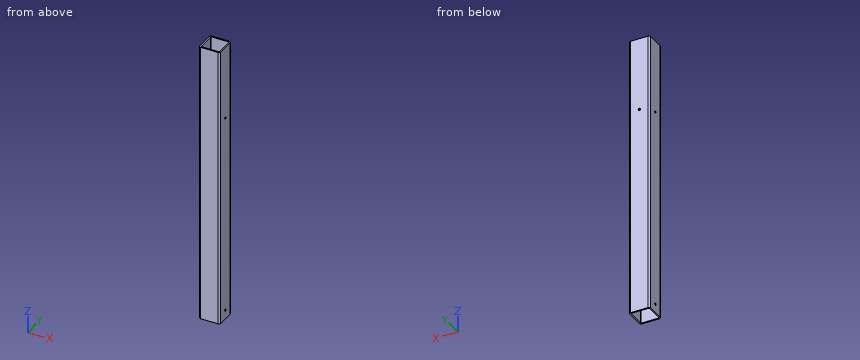
Autodesk Inventor part; units mm, degrees
ref_plane "YZ Plane" through (0, 0, 0) normal (1, 0, 0) x (0, 1, 0)
ref_plane "XZ Plane" through (0, 0, 0) normal (0, 1, 0) x (-1, 0, 0)
ref_plane "XY Plane" through (0, 0, 0) normal (0, 0, 1) x (1, 0, 0)
sketch "Sketch1" plane through (0, 0, 0) normal (0, 0, 1) x (1, 0, 0)
  line L0 (40, 34) -> (40, -34)
  line L1 (34, -40) -> (-34, -40)
  line L2 (-40, -34) -> (-40, 34)
  line L3 (-34, 40) -> (34, 40)
  arc A0 (-34, 40) -> (-40, 34) centre (-34, 34) ccw
  arc A1 (40, 34) -> (34, 40) centre (34, 34) ccw
  arc A2 (34, -40) -> (40, -34) centre (34, -34) ccw
  arc A3 (-40, -34) -> (-34, -40) centre (-34, -34) ccw
  arc A4 (-34, 35) -> (-35, 34) centre (-34, 34) ccw
  line L4 (-34, 35) -> (34, 35)
  arc A5 (35, 34) -> (34, 35) centre (34, 34) ccw
  line L5 (35, 34) -> (35, -34)
  arc A6 (34, -35) -> (35, -34) centre (34, -34) ccw
  line L6 (34, -35) -> (-34, -35)
  arc A7 (-35, -34) -> (-34, -35) centre (-34, -34) ccw
  line L7 (-35, -34) -> (-35, 34)
  point P0 (0, 0)
  point P1 (0, 0)
  point P2 (40, 40)
  point P3 (40, -40)
  point P4 (-40, -40)
  point P5 (-40, 40)
  dimension "d0" = 80
  dimension "d1" = 6
  dimension "d2" = 5
extrude "Extrusion1" add sketch "Sketch1" along normal blind 1094
sketch "Sketch2" plane through (40, -34, 0) normal (1, 0, 0) x (0, 0, -1)
  line L0 (0, 0) -> (-1094, 0)
  line L1 (0, 68) -> (0, 0)
  point P0 (-809, 34)
  point P1 (-35, 34)
  dimension "d5" = 809
  dimension "d6" = 34
  dimension "d15" = 35
hole "Hole1" at (40, 0, 809) at (40, 0, 35) direction (-1, 0, 0) diameter 9 end through all
sketch "Sketch3" plane through (-34, 40, 0) normal (0, 1, 0) x (1, 0, 0)
  line L0 (68, 0) -> (68, -1094)
  line L1 (0, 0) -> (68, 0)
  point P0 (34, -809)
  dimension "d16" = 34
  dimension "d17" = 809
hole "Hole2" at (0, 40, 809) direction (0, -1, 0) diameter 9 depth 8 tip angle 118
properties part number "3136 1094 48" material "Steel, Mild"
CAD build for the part. Positions are in the model's coordinates, mm. Coordinates: 2 decimals unless noted, no trailing zeros. Write each loop counter-clockwise with the first axis right and the second up, starting at its lowest first coordinate (ties: lowest second). Pieces come first, ordered by that corner, then holes. Notation, with made-up numbers: (34.5, 80.5) -> (64.5, 80.5) arc R13 ccw to (64.5, 84.5) -> close; hole circle Ø9 at (45, 57.25). An arc over 180 degrees is marked (long way). Return JSON: item names as keys, results as strings. Group by question number.
Q1. Flat gauge pin, fed straight in: pin 1 (11.5 mm diameter, centred on x = 0, z = 809, fed in from +Y). Where does the tip first touch, or does it go through?
Q2. Cut at B-B, the plane x = 16. Give the cut face in (y, z), then the cut area to 3 significant figures.
Q3. Cut at A-A, the plane z = 505.5. Give the cut face in (x, y), then the cut area to 3 significant figures.
Q4. Drill centre lines: line 1 (Z direction, x = -37.85, y = 0); line 2 (X direction, y = -23.5, z = 498.5). Where is each one in solid material? Low to high.
Returned:
{
 "1": {"pin 1": "stops at y = 40"},
 "2": {"outline": "(-40, 0) -> (-35, 0) -> (-35, 1094) -> (-40, 1094) -> close; (35, 0) -> (40, 0) -> (40, 1094) -> (35, 1094) -> close", "area": "10,900 mm2"},
 "3": {"outline": "(-40, -34) arc R6 ccw to (-34, -40) -> (34, -40) arc R6 ccw to (40, -34) -> (40, 34) arc R6 ccw to (34, 40) -> (-34, 40) arc R6 ccw to (-40, 34) -> close; hole (-35, -34) arc R1 ccw to (-34, -35) -> (34, -35) arc R1 ccw to (35, -34) -> (35, 34) arc R1 ccw to (34, 35) -> (-34, 35) arc R1 ccw to (-35, 34) -> close", "area": "1,470 mm2"},
 "4": {"line 1": "z = 0 to 30.5, 39.5 to 804.5, 813.5 to 1094", "line 2": "x = -40 to -35, 35 to 40"}
}
